Read the model definition and answer for the solid it produces. Units are mm, in the model's axes. Face numbers are marked on the shaded views. A direction names the side the tool comes from. Coordinates: 2 decimals unless noted, no trailing zeros. Loops run counter-clockwise (first coordinate to the right, second up) from the corner with the lowest first, then second, coordinate; pieces in that order, holes last. Notation, with made-up numbers: (19.25, 25) - (24.25, 25) arc R33 ccw to (24.25, 57) - close; hole circle Ø4 at (23, 62.5). An arc over 180 degrees is marked (long way). Use one line per item in the form item = value. Start each with the question number.
1) Consider line 1 (Z direction, x = 4, y = -13); line 2 (Z direction, x = -3.5, y = -16); line 3 (Z direction, x = 7, y = -3.5). Determine where each line is inside the solid, lowest interval first.
2) A cutting plane is placed at A-A (z = 2.5). Give the vertices of the cut face in (x, y).
3) A cutting plane is placed at B-B (x = -3.25). Give the vertices of the cut face in (y, z), and give its area (3 significant figures).
4) A cutting plane is placed at D-D (x = 0.75). Give the vertices of the cut face in (y, z).
5) The mould has two halves that part along Z. Classify the marked faces 1, 2 and 3: released by +Z, released by -Z, zero draft, split by the parting line, or undercut.
6) Each of these flat-tipped pins is pushed along its axis until it touches: P1, Ø3.5, axis at x = -7.5, y = 1, coming from the +Z side; P2, Ø1, axis at y = -25, z = 28.5, coming from the -X side; P3, Ø4.5, axis at x = 2.5, z = 29, coming from the -Y side. Where does it stop, or does it pass through?
7) Which of the six approach directions +Z, -Z, +X, -X, +Y, -Y give full straight-line access (tool end or side, diameter ignored) to the marked faces 4, 5 and 6?
8) A cutting plane is placed at C-C (y = 0.5). Give the vertices of the cut face in (x, z), and give its area (3 significant figures).
from build123d import *

# Parameters (mm, degrees)
F1_DEPTH   = 10
F2_DEPTH   = 10
F4_DEPTH   = 30
F5_DEPTH   = 4
F4_FACE1_W = 5.5
F4_FACE1_H = 26


with BuildPart() as f1:
    # F0 (on Right) → F1 (new body)
    with BuildSketch(Plane.YZ):
        with BuildLine():
            Line((0, 0), (-30, 0))
            Line((-30, 0), (-30, 4))
            ThreePointArc((-30, 4), (-22.698520979, 22.698520979), (-4, 30))
            Line((-4, 30), (0, 30))
            Line((0, 30), (0, 26))
            Line((0, 26), (4, 30))
            Line((4, 30), (4, 34))
            Line((4, 34), (0, 34))
            Line((0, 34), (-4, 34))
            ThreePointArc((-4, 34), (-25.2132034356, 25.2132034356), (-34, 4))
            Line((-34, 4), (-34, -4))
            Line((-34, -4), (-30, -4))
            Line((-30, -4), (0, -4))
            Line((0, -4), (4, -4))
            Line((4, -4), (4, 0))
            Line((4, 0), (0, 4))
            Line((0, 4), (0, 0))
        make_face()
    extrude(amount=-F1_DEPTH)

    # F2 (add): a face of the model
    f2_faces = [f1.faces().sort_by_distance(p)[0] for p in [
        (0, 3.4625988463, 32),
    ]]
    extrude(f2_faces, amount=F2_DEPTH)

    # F3 (on Front) → F4 (join)
    with BuildSketch(Plane.XZ):
        Polygon((0, 34), (2.75, 34), (2.75, 36), (5.25, 36), (5.25, 37.75), (2.75, 40.25), (-2.75, 40.25), (-5.25, 37.75), (-5.25, 36), (-2.75, 36), (-2.75, 34), align=None)
    extrude(amount=F4_DEPTH)

    # F5 (add): a face of the model
    f5_faces = [f1.faces().sort_by_distance(p)[0] for p in [
        (0, 0, 37.2652953586),
    ]]
    extrude(f5_faces, amount=F5_DEPTH)

    # F4_face1 (on face) → F6 (join, up to the next surface of F1)
    with BuildSketch(Plane(origin=(0, -17, 34), x_dir=(1, 0, 0), z_dir=(0, 0, -1))):
        Rectangle(F4_FACE1_W, F4_FACE1_H)
    extrude(until=Until.NEXT)


solid = f1.part
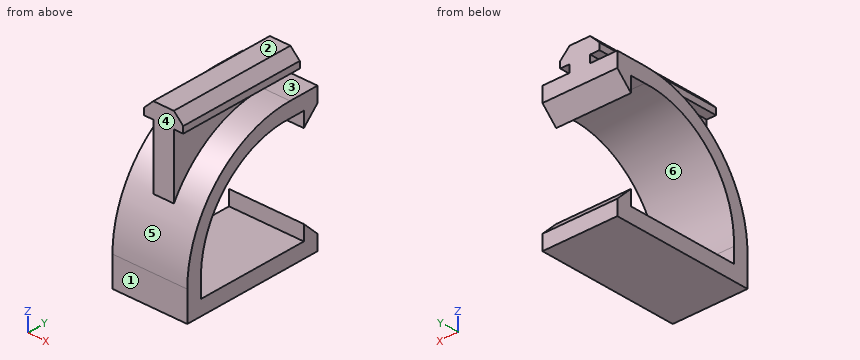
Found:
q1.line_1 = -4 to 0, 28.71 to 32.62, 36 to 39
q1.line_2 = -4 to 0, 27.48 to 31.5, 36 to 39.5
q1.line_3 = -4 to 0, 30 to 34
q2.outline = (-10, -34) - (10, -34) - (10, -30) - (-10, -30) - close; (-10, 0) - (10, 0) - (10, 1.5) - (-10, 1.5) - close
q3.outline = (-34, -4) - (4, -4) - (4, 0) - (0, 4) - (0, 0) - (-30, 0) - (-30, 4) arc R25 cw to (-4, 30) - (0, 30) - (0, 26) - (4, 30) - (4, 34) - (-4, 34) arc R30 ccw to (-34, 4) - close; (-30, 36) - (4, 36) - (4, 39.75) - (-30, 39.75) - close
q3.area = 507 mm^2
q4.outline = (-34, -4) - (4, -4) - (4, 0) - (0, 4) - (0, 0) - (-30, 0) - (-30, 4) arc R25 cw to (-4, 30) - (0, 30) - (0, 26) - (4, 30) - (4, 40.25) - (-30, 40.25) - (-30, 18.97) arc R30 ccw to (-34, 4) - close
q5.face_1 = zero draft
q5.face_2 = released by +Z
q5.face_3 = undercut
q6.P1 = 34
q6.P2 = -2.75
q6.P3 = -30
q7.face_4 = +Z, +X, -X, -Y
q7.face_5 = -Y
q7.face_6 = +X, -X
q8.outline = (-10, -4) - (10, -4) - (10, 3.5) - (-10, 3.5) - close; (-10, 26.5) - (10, 26.5) - (10, 34) - (2.75, 34) - (2.75, 36) - (5.25, 36) - (5.25, 37.75) - (2.75, 40.25) - (-2.75, 40.25) - (-5.25, 37.75) - (-5.25, 36) - (-2.75, 36) - (-2.75, 34) - (-10, 34) - close
q8.area = 349 mm^2
